from build123d import *

# Parameters (mm, degrees)
SKETCH1_W             = 18.5
SKETCH1_H             = 18.5
BOSS_EXTRUDE1_DEPTH   = 5
BOSS_EXTRUDE1_2_DEPTH = 5
BOSS_EXTRUDE1_3_DEPTH = 5
BOSS_EXTRUDE1_4_DEPTH = 5
BOSS_EXTRUDE2_DEPTH   = 88.9
SKETCH3_R             = 3.2
BOSS_EXTRUDE3_DEPTH   = 20
BOSS_EXTRUDE4_DEPTH   = 7.5
FILLET1_R             = 3
SKETCH5_W             = 94.9
SKETCH5_H             = 94.9
CUT_EXTRUDE1_DEPTH    = 4.2
CUT_EXTRUDE2_DEPTH    = 5


with BuildPart() as part:
    # Sketch1 → Boss-Extrude1 (new body)
    with BuildSketch(Plane(origin=(0, 0, 0), x_dir=(1, 0, 0), z_dir=(0, 1, 0))):
        with Locations((-62.75, 62.75)):
            Rectangle(SKETCH1_W, SKETCH1_H)
    extrude(amount=BOSS_EXTRUDE1_DEPTH)



with BuildPart() as body_2:
    # Sketch1 → Boss-Extrude1 2 (new body)
    with BuildSketch(Plane(origin=(0, 0, 0), x_dir=(1, 0, 0), z_dir=(0, 1, 0))):
        with Locations((-62.75, -62.75)):
            Rectangle(SKETCH1_W, SKETCH1_H)
    extrude(amount=BOSS_EXTRUDE1_2_DEPTH)


with BuildPart() as body_3:
    # Sketch1 → Boss-Extrude1 3 (new body)
    with BuildSketch(Plane(origin=(0, 0, 0), x_dir=(1, 0, 0), z_dir=(0, 1, 0))):
        with Locations((62.75, -62.75)):
            Rectangle(SKETCH1_W, SKETCH1_H)
    extrude(amount=BOSS_EXTRUDE1_3_DEPTH)


with BuildPart() as body_4:
    # Sketch1 → Boss-Extrude1 4 (new body)
    with BuildSketch(Plane(origin=(0, 0, 0), x_dir=(1, 0, 0), z_dir=(0, 1, 0))):
        with Locations((62.75, 62.75)):
            Rectangle(SKETCH1_W, SKETCH1_H)
    extrude(amount=BOSS_EXTRUDE1_4_DEPTH)


with BuildPart() as part_1:
    add(part.part)

    add(body_2.part)  # Boss-Extrude2 merges body 2

    add(body_3.part)  # Boss-Extrude2 merges body 3

    add(body_4.part)  # Boss-Extrude2 merges body 4
    # Sketch2 → Boss-Extrude2 (add)
    with BuildSketch(Plane.XZ):
        Polygon((-72, -53.5), (-72, -48.5), (-48.5, -48.5), (-48.5, -72), (-53.5, -72), (-53.5, -53.5), align=None)
        Polygon((-72, 53.5), (-53.5, 53.5), (-53.5, 72), (-48.5, 72), (-48.5, 48.5), (-72, 48.5), align=None)
        Polygon((72, -53.5), (53.5, -53.5), (53.5, -72), (48.5, -72), (48.5, -48.5), (72, -48.5), align=None)
        Polygon((72, 53.5), (72, 48.5), (48.5, 48.5), (48.5, 72), (53.5, 72), (53.5, 53.5), align=None)
    extrude(amount=-BOSS_EXTRUDE2_DEPTH)

    # Sketch3 → Boss-Extrude3 (add)
    with BuildSketch(Plane.XZ):
        with Locations(Location((-63.75, 63.75, 0), (0, 0, 270))):
            Circle(SKETCH3_R)
        with Locations(Location((63.75, 63.75, 0), (0, 0, 270))):
            Circle(SKETCH3_R)
        with Locations(Location((-63.75, -63.75, 0), (0, 0, 90))):
            Circle(SKETCH3_R)
        with Locations(Location((63.75, -63.75, 0), (0, 0, 90))):
            Circle(SKETCH3_R)
    extrude(amount=BOSS_EXTRUDE3_DEPTH)

    # Sketch4 → Boss-Extrude4 (add)
    with BuildSketch(Plane(origin=(0, 88.9, 0), x_dir=(1, 0, 0), z_dir=(0, 1, 0))):
        Polygon((-72, 53.5), (-72, -53.5), (-53.5, -53.5), (-53.5, -72), (53.5, -72), (53.5, -53.5), (72, -53.5), (72, 53.5), (53.5, 53.5), (53.5, 72), (-53.5, 72), (-53.5, 53.5), align=None)
    extrude(amount=BOSS_EXTRUDE4_DEPTH)

    # Fillet1
    fillet1_edges = [part_1.edges().sort_by_distance(p)[0] for p in [
        (-62.75, 96.4, -53.5),
        (-72, 96.4, 0),
        (-62.75, 96.4, 53.5),
        (-53.5, 96.4, 62.75),
        (0, 96.4, 72),
        (53.5, 96.4, 62.75),
        (62.75, 96.4, 53.5),
        (72, 96.4, 0),
        (62.75, 96.4, -53.5),
        (53.5, 96.4, -62.75),
        (0, 96.4, -72),
        (-53.5, 96.4, -62.75),
    ]]
    fillet(fillet1_edges, radius=FILLET1_R)

    # Sketch5 → Cut-Extrude1 (cut)
    with BuildSketch(Plane(origin=(0, 96.4, 0), x_dir=(1, 0, 0), z_dir=(0, 1, 0))):
        Rectangle(SKETCH5_W, SKETCH5_H)
    extrude(amount=-CUT_EXTRUDE1_DEPTH, mode=Mode.SUBTRACT)

    # Sketch6 → Cut-Extrude2 (cut)
    with BuildSketch(Plane(origin=(0, 96.4, 0), x_dir=(1, 0, 0), z_dir=(0, 1, 0))):
        with BuildLine():
            Line((-47.45, 10), (47.45, 10))
            ThreePointArc((47.45, 10), (57.45, 0), (47.45, -10))
            Line((47.45, -10), (-47.45, -10))
            ThreePointArc((-47.45, -10), (-57.45, 0), (-47.45, 10))
        make_face()
    extrude(amount=-CUT_EXTRUDE2_DEPTH, mode=Mode.SUBTRACT)


solid = part_1.part
Can you work these out from the model? Positions are in its coordinate system, mm. A direction names the side the tool comes from. Round coordinates to 2 decimals unless told otherwise and drop trailing zeros. Order: outer loops, then holes, each group sorted by start corner. A loop starts at its lowest first (then second) coordinate and runs counter-clockwise, first axis right, second up. Notation, with made-up numbers: M -7,15.5 L 1,15.5 A14 ccw 1,37.5 Z; hole C 35.5,51.25 d11. An arc over 180 degrees is marked long. Use a Markdown table: item, result.
1) On a 3-axis mill with a long thin cutter (end or side, diameter ignored), from which of +Z, -Z, +X, -X, +Y, -Y can I reach the whole of each face in a straight line? I mean faces 1 (the face through (-63, 49, 53.5)), 2 (the face through (-60, 0, 60)), 3 (the face through (48.5, 44, 60)). Say none if no direction works.
Geometry says:
| item | result |
|---|---|
| face 1 | +Z, -X, +Y |
| face 2 | -Y |
| face 3 | +Z, -Z, -Y |
2) If we mould it in two halves opening along X, with no side actions, what happens to faces 4 (the face through (-72, 50, 53)), 5 (the face through (72, 50, -53)), 6 (the face through (-1, 88.9, -1)), 7 (the face through (-60, 44, -48.5))? For each: +X half, -X half, draft (parallel to the pull), parting line (faces both ways), or undercut.
Geometry says:
| item | result |
|---|---|
| face 4 | -X half |
| face 5 | +X half |
| face 6 | undercut |
| face 7 | draft |
3) Imagine slicing it at D-D (z = 34). List the corners of the cut face in (x, y) for me.
Geometry says:
| item | result |
|---|---|
| outline | M -72,88.9 L 72,88.9 L 72,93.4 A3 ccw 69,96.4 L 47.45,96.4 L 47.45,92.2 L -47.45,92.2 L -47.45,96.4 L -69,96.4 A3 ccw -72,93.4 Z |
4) Imagine slicing it at B-B (z = 63.75). List the corners of the cut face in (x, y) for me.
Geometry says:
| item | result |
|---|---|
| outline | M -72,0 L -66.95,0 L -66.95,-20 L -60.55,-20 L -60.55,0 L -48.5,0 L -48.5,88.9 L 48.5,88.9 L 48.5,0 L 60.55,0 L 60.55,-20 L 66.95,-20 L 66.95,0 L 72,0 L 72,5 L 53.5,5 L 53.5,93.4 A3 ccw 50.5,96.4 L -50.5,96.4 A3 ccw -53.5,93.4 L -53.5,5 L -72,5 Z |
5) Imagine slicing it at A-A (y = 84). List the corners of the cut face in (x, z) for me.
Geometry says:
| item | result |
|---|---|
| outline | M -72,-53.5 L -53.5,-53.5 L -53.5,-72 L -48.5,-72 L -48.5,-48.5 L -72,-48.5 Z; M -72,48.5 L -48.5,48.5 L -48.5,72 L -53.5,72 L -53.5,53.5 L -72,53.5 Z; M 48.5,-72 L 53.5,-72 L 53.5,-53.5 L 72,-53.5 L 72,-48.5 L 48.5,-48.5 Z; M 48.5,48.5 L 72,48.5 L 72,53.5 L 53.5,53.5 L 53.5,72 L 48.5,72 Z |
6) I'm going to push flat-ended pins straight in: P1, Ø15, axis at x = -63.5, y = 52.5, coming from the +Z side; P2, Ø3, axis at x = -5.5, z = -24, coming from the -Y side; P3, Ø7, axis at x = 56.5, z = 58, coming from the -Y side. Where does each tip first touch, or does it pass through?
Geometry says:
| item | result |
|---|---|
| P1 | stops at z = 53.5 |
| P2 | stops at y = 88.9 |
| P3 | stops at y = 0 |
7) If I drill on line 1 along Z through (x, y) = (-54, 29.5); line 2 along X through (y, z) = (1, -54.5), over which ranges is the centre line in solid material (lowest first)?
Geometry says:
| item | result |
|---|---|
| line 1 | z = -53.5 to -48.5, 48.5 to 53.5 |
| line 2 | x = -72 to -48.5, 48.5 to 72 |
8) Imagine slicing it at C-C (x = 63.75). List the corners of the cut face in (y, z) for me, then the cut area to 3 significant figures.
Geometry says:
| item | result |
|---|---|
| outline | M -20,-66.95 L 0,-66.95 L 0,-72 L 5,-72 L 5,-53.5 L 93.4,-53.5 A3 ccw 96.4,-50.5 L 96.4,50.5 A3 ccw 93.4,53.5 L 5,53.5 L 5,72 L 0,72 L 0,66.95 L -20,66.95 L -20,60.55 L 0,60.55 L 0,48.5 L 88.9,48.5 L 88.9,-48.5 L 0,-48.5 L 0,-60.55 L -20,-60.55 Z |
| area | 2,130 mm² |
